Part model, mm, in its own coordinate system. Face numbers are marked on the shaded views. A direction names the side the tool comes from. Round coordinates to 2 decimals unless told otherwise and drop trailing zeros. Write each loop counter-clockwise with the first axis right and the second up, starting at its lowest first coordinate (ties: lowest second). Pieces come first, ordered by that corner, then holes. Notation, with made-up numbers: (78, -5) -> (118, -5) arc R14 ccw to (118, 6) -> close; hole circle Ø7 at (-1, 78.25). An arc over 180 degrees is marked (long way). Return JSON: item names as keys, results as strings. Group by question number.
(1) Tool access for the marked faces 1, 2, 3 and 4: list every direction of +Z, -Z, +X, -X, +Y, -Y with a clear straight run to the whole face (end or side of a thin tool).
(2) Saw through at D-D (y = 36). List the corners of the cut face in (x, z).
(3) Drop flat-ended pins along their axis: pin 1 Ø0.8 at (x, y) = (6, 14) entering from -Z; pin 2 Ø3 at (x, z) = (3, -22) entering from +Y; pin 3 Ø2.5 at (x, y) = (4, 25.5) entering from +Z. Give the stop position or say it passes through.
(4) Drill centre lines: L1, parallel to Y at x = 5.75, z = -18; L2, parallel to Y at x = 4, z = -15.5; L3, parallel to Y at x = 1, z = -25.5. Where is each one in solid material? Low to high. Write a range as from..to.
(5) Saw through at A-A (z = -18). List the corners of the cut face in (x, y), plus the area to 3 significant figures.
(6) Saw through at C-C (z = -26). List the corners of the cut face in (x, y).
(7) Mould opens along Y. For the marked faces 5, 6, 7 and 8 say: +Y half, -Y half, draft (parallel to the pull), parting line (faces both ways), or undercut.
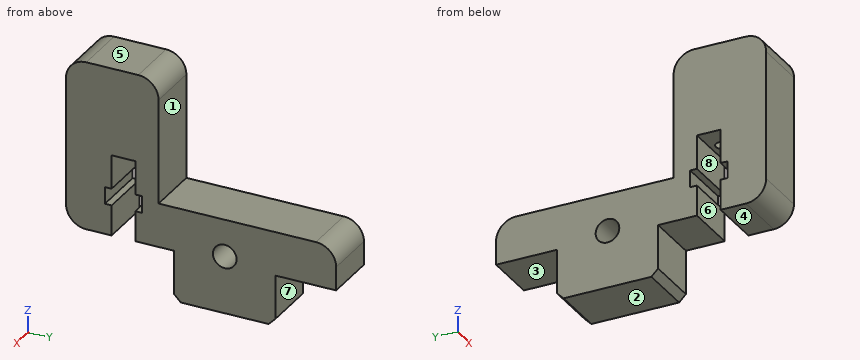
from build123d import *

# Parameters (mm, degrees)
SKETCH1_R      = 1.75
EXTRUDE1_DEPTH = 8
SKETCH2_R      = 1
EXTRUDE2_DEPTH = 1


with BuildPart() as part:
    # Sketch1 → Extrude1 (new body)
    with BuildSketch(Plane(origin=(0, 0, 0), x_dir=(0, 0, -1), z_dir=(1, 0, 0))):
        with BuildLine():
            Line((28.082940188, 19.097217002), (34.582940188, 19.097217002))
            Line((34.582940188, 19.097217002), (35.582940188, 20.097217002))
            Line((35.582940188, 20.097217002), (35.582940188, 33.097217002))
            Line((35.582940188, 33.097217002), (34.582940188, 34.097217002))
            Line((34.582940188, 34.097217002), (28.082940188, 34.097217002))
            Line((28.082940188, 34.097217002), (28.082940188, 43.097217002))
            Line((28.082940188, 43.097217002), (24.582940188, 43.097217002))
            ThreePointArc((24.582940188, 43.097217002), (22.461619844, 42.218537346), (21.582940188, 40.097217002))
            Line((21.582940188, 40.097217002), (21.582940188, 16.797217002))
            Line((21.582940188, 16.797217002), (6.082940188, 16.797217002))
            ThreePointArc((6.082940188, 16.797217002), (3.961619844, 15.918537346), (3.082940188, 13.797217002))
            Line((3.082940188, 13.797217002), (3.082940188, 6.097217002))
            ThreePointArc((3.082940188, 6.097217002), (3.961619844, 3.975896659), (6.082940188, 3.097217002))
            Line((6.082940188, 3.097217002), (25.082940188, 3.097217002))
            ThreePointArc((25.082940188, 3.097217002), (27.204260531, 3.975896659), (28.082940188, 6.097217002))
            Line((28.082940188, 6.097217002), (28.082940188, 9.847217002))
            Line((28.082940188, 9.847217002), (23.582940188, 9.847217002))
            Line((23.582940188, 9.847217002), (23.582940188, 8.847217002))
            Line((23.582940188, 8.847217002), (21.082940188, 8.847217002))
            Line((21.082940188, 8.847217002), (21.082940188, 9.847217002))
            Line((21.082940188, 9.847217002), (16.082940188, 9.847217002))
            Line((16.082940188, 9.847217002), (16.082940188, 13.347217002))
            Line((16.082940188, 13.347217002), (21.082940188, 13.347217002))
            Line((21.082940188, 13.347217002), (21.082940188, 14.347217002))
            Line((21.082940188, 14.347217002), (23.582940188, 14.347217002))
            Line((23.582940188, 14.347217002), (23.582940188, 13.347217002))
            Line((23.582940188, 13.347217002), (28.082940188, 13.347217002))
            Line((28.082940188, 13.347217002), (28.082940188, 19.097217002))
        make_face()
        with Locations((27.082940188, 26.597217002)):
            Circle(SKETCH1_R, mode=Mode.SUBTRACT)
    extrude(amount=EXTRUDE1_DEPTH)

    # Sketch2 → Extrude2 (cut)
    with BuildSketch(Plane(origin=(0, 0, -16.082940188), x_dir=(-1, 0, 0), z_dir=(0, 0, -1))):
        with Locations((-4, 11.597217002)):
            Circle(SKETCH2_R)
    extrude(amount=-EXTRUDE2_DEPTH, mode=Mode.SUBTRACT)


solid = part.part
Computed values:
{
 "1": {"face 1": "+Z, +X, -X, +Y", "face 2": "-Z, +X, -X, +Y, -Y", "face 3": "-Z, +X, -X, +Y", "face 4": "-Z, +X, -X, -Y"},
 "2": {"outline": "(0, -28.08) -> (8, -28.08) -> (8, -21.58) -> (0, -21.58) -> close"},
 "3": {"pin 1": "z = -28.08", "pin 2": "y = 42.89", "pin 3": "z = -21.58"},
 "4": {"L1": "3.1..9.85, 13.35..16.8", "L2": "3.1..10.6, 12.6..16.8", "L3": "3.13..9.85, 13.35..25.85, 27.34..43.1"},
 "5": {"outline": "(0, 3.1) -> (8, 3.1) -> (8, 9.85) -> (0, 9.85) -> close; (0, 13.35) -> (8, 13.35) -> (8, 16.8) -> (0, 16.8) -> close", "area": "81.6 mm2"},
 "6": {"outline": "(0, 3.24) -> (8, 3.24) -> (8, 9.85) -> (0, 9.85) -> close; (0, 13.35) -> (8, 13.35) -> (8, 25.22) -> (0, 25.22) -> close; (0, 27.97) -> (8, 27.97) -> (8, 43.1) -> (0, 43.1) -> close"},
 "7": {"face 5": "draft", "face 6": "undercut", "face 7": "+Y half", "face 8": "undercut"}
}
